Work out the finished part from the listing and answer in its coordinate system (mm). Give positions to 0.01 mm unless a question says otherwise; leave off trailing zeros. Loops run counter-clockwise (first coordinate to the right, second up) from the corner with the lowest first, then second, coordinate; pieces in that order, holes last.
```python
from build123d import *

# Parameters (mm, degrees)
F1_DEPTH = 3.175


with BuildPart() as f1:
    # F0 (on Top) → F1 (new body)
    with BuildSketch(Plane.XY):
        with BuildLine():
            ThreePointArc((28.922397, -102.872733), (41.462552, -98.040783), (52.705, -90.678))
            Line((52.705, -90.678), (52.705, 31.242))
            add(Edge.make_bspline(
                [(52.705, 31.242), (52.705, 50.292), (61.6839, 44.958), (70.0659, 50.8)],
                knots=[0, 0, 0, 0, 26.151792, 26.151792, 26.151792, 26.151792], degree=3))
            ThreePointArc((70.0659, 50.8), (63.662757, 67.803409), (49.909777, 79.676559))
            ThreePointArc((49.909777, 79.676559), (25.638664, 88.459394), (0, 91.44))
            ThreePointArc((0, 91.44), (-25.638664, 88.459394), (-49.909777, 79.676559))
            ThreePointArc((-49.909777, 79.676559), (-63.662757, 67.803409), (-70.0659, 50.8))
            add(Edge.make_bspline(
                [(-52.705, 31.242), (-52.705, 50.292), (-61.6839, 44.958), (-70.0659, 50.8)],
                knots=[0, 0, 0, 0, 26.151792, 26.151792, 26.151792, 26.151792], degree=3))
            Line((-52.705, 31.242), (-52.705, -90.678))
            ThreePointArc((-52.705, -90.678), (-41.462552, -98.040783), (-28.922397, -102.872733))
            ThreePointArc((-28.922397, -102.872733), (-14.585955, -105.724095), (0, -106.68))
            ThreePointArc((0, -106.68), (14.585955, -105.724095), (28.922397, -102.872733))
        make_face()
    extrude(amount=F1_DEPTH)


solid = f1.part
```
Q1. Given pin 1 (1 mm diameter, centred on y = -39, z = 1, fed in from +X) (3 decimals); pin 2 (1 mm diameter, centred on y = 34.5, z = 0.5, fed in from +X); pin 3 (1 mm diameter, centred on y = -0.5, z = 2, fed in from -X) (3 decimals), each flat-ended and moving along its own axis, determine where each tip first touches the part or whether it passes through.
Q2. Section B-B on x = -35 is taken. Give the vertices of the cut face in (y, z) (3 decimals).
Q3. Consider line 1 along Y through (x, z) = (1.5, 0.3); line 2 along X through (y, z) = (-57.5, 2.05) (3 decimals); line 3 along X through (y, z) = (-95, 1.4). Determine where each line is inside the solid, lowest interval first.
Q4. Section A-A on y = -25 is taken. Give the vertices of the cut face in (x, z) (3 decimals).
Check result:
1. pin 1: stops at x = 52.705
1. pin 2: stops at x = 52.84
1. pin 3: stops at x = -52.705
2. outline: (-100.912, 0) - (85.818, 0) - (85.818, 3.175) - (-100.912, 3.175) - close
3. line 1: y = -106.67 to 91.43
3. line 2: x = -52.705 to 52.705
3. line 3: x = -46.75 to 46.75
4. outline: (-52.705, 0) - (52.705, 0) - (52.705, 3.175) - (-52.705, 3.175) - close
